```python
from build123d import *

# Parameters (mm, degrees)
SKETCH_281X300_25_R   = 1.6
SKETCH_281X300_25_R_2 = 15
SKETCH_281X300_25_R_3 = 2.15
SKETCH_281X300_25_R_4 = 2.2
SKETCH_281X300_25_W   = 73
SKETCH_281X300_25_H   = 40
F_4MM_DEPTH           = 4
FILLET_1_R            = 8


with BuildPart() as part:
    # Sketch 281x300__25 → 4mm (new body)
    with BuildSketch(Plane.XY):
        Polygon((-51, 150), (53, 150), (53, 100), (137.5, 100), (137.5, -100), (53, -100), (53, -150), (-51, -150), (-51, -100), (-135.5, -100), (-135.5, 100), (-51, 100), align=None)
        with Locations((84.5, -60)):
            Circle(SKETCH_281X300_25_R, mode=Mode.SUBTRACT)
        with Locations((114.5, -60)):
            Circle(SKETCH_281X300_25_R, mode=Mode.SUBTRACT)
        with Locations((84.5, 61)):
            Circle(SKETCH_281X300_25_R, mode=Mode.SUBTRACT)
        with Locations((1, 90.5)):
            Circle(SKETCH_281X300_25_R_2, mode=Mode.SUBTRACT)
        with Locations((1, 125)):
            Circle(SKETCH_281X300_25_R_3, mode=Mode.SUBTRACT)
        with Locations((-33.5, 90.5)):
            Circle(SKETCH_281X300_25_R_3, mode=Mode.SUBTRACT)
        with Locations((35.5, 90.5)):
            Circle(SKETCH_281X300_25_R_3, mode=Mode.SUBTRACT)
        with Locations((-44, 140)):
            Circle(SKETCH_281X300_25_R_3, mode=Mode.SUBTRACT)
        with Locations((114.5, 61)):
            Circle(SKETCH_281X300_25_R, mode=Mode.SUBTRACT)
        with Locations((1, 56)):
            Circle(SKETCH_281X300_25_R_3, mode=Mode.SUBTRACT)
        with Locations((26, -140)):
            Circle(SKETCH_281X300_25_R_4, mode=Mode.SUBTRACT)
        with Locations((-24, -140)):
            Circle(SKETCH_281X300_25_R_4, mode=Mode.SUBTRACT)
        with Locations((-24, -90)):
            Circle(SKETCH_281X300_25_R_4, mode=Mode.SUBTRACT)
        with Locations((26, -90)):
            Circle(SKETCH_281X300_25_R_4, mode=Mode.SUBTRACT)
        with Locations((1, 111.5)):
            Circle(SKETCH_281X300_25_R, mode=Mode.SUBTRACT)
        with Locations((84.5, -90)):
            Circle(SKETCH_281X300_25_R, mode=Mode.SUBTRACT)
        with Locations((84.5, 91)):
            Circle(SKETCH_281X300_25_R, mode=Mode.SUBTRACT)
        with Locations((114.5, 91)):
            Circle(SKETCH_281X300_25_R, mode=Mode.SUBTRACT)
        with Locations((114.5, -90)):
            Circle(SKETCH_281X300_25_R, mode=Mode.SUBTRACT)
        with Locations((118.5, 10)):
            Circle(SKETCH_281X300_25_R, mode=Mode.SUBTRACT)
        with Locations((118.5, -10)):
            Circle(SKETCH_281X300_25_R, mode=Mode.SUBTRACT)
        with Locations((-120.5, 10)):
            Circle(SKETCH_281X300_25_R, mode=Mode.SUBTRACT)
        with Locations((-120.5, -10)):
            Circle(SKETCH_281X300_25_R, mode=Mode.SUBTRACT)
        with Locations((-115.5, -91)):
            Circle(SKETCH_281X300_25_R, mode=Mode.SUBTRACT)
        with Locations((-85.5, -91)):
            Circle(SKETCH_281X300_25_R, mode=Mode.SUBTRACT)
        with Locations((-115.5, 91)):
            Circle(SKETCH_281X300_25_R, mode=Mode.SUBTRACT)
        with Locations((-85.5, 91)):
            Circle(SKETCH_281X300_25_R, mode=Mode.SUBTRACT)
        with Locations((-85.5, 61)):
            Circle(SKETCH_281X300_25_R, mode=Mode.SUBTRACT)
        with Locations((-115.5, 61)):
            Circle(SKETCH_281X300_25_R, mode=Mode.SUBTRACT)
        with Locations((-85.5, -61)):
            Circle(SKETCH_281X300_25_R, mode=Mode.SUBTRACT)
        with Locations((-115.5, -61)):
            Circle(SKETCH_281X300_25_R, mode=Mode.SUBTRACT)
        with Locations((118.5, 43)):
            Circle(SKETCH_281X300_25_R, mode=Mode.SUBTRACT)
        with Locations((118.5, -42)):
            Circle(SKETCH_281X300_25_R, mode=Mode.SUBTRACT)
        with Locations((-120.5, 43)):
            Circle(SKETCH_281X300_25_R, mode=Mode.SUBTRACT)
        with Locations((46, 140)):
            Circle(SKETCH_281X300_25_R_3, mode=Mode.SUBTRACT)
        with Locations((-44, -140)):
            Circle(SKETCH_281X300_25_R_3, mode=Mode.SUBTRACT)
        with Locations((46, -140)):
            Circle(SKETCH_281X300_25_R_3, mode=Mode.SUBTRACT)
        with Locations((19.186533479, 101)):
            Circle(SKETCH_281X300_25_R, mode=Mode.SUBTRACT)
        with Locations((19.186533479, 80)):
            Circle(SKETCH_281X300_25_R, mode=Mode.SUBTRACT)
        with Locations((1, 69.5)):
            Circle(SKETCH_281X300_25_R, mode=Mode.SUBTRACT)
        with Locations((-17.186533479, 80)):
            Circle(SKETCH_281X300_25_R, mode=Mode.SUBTRACT)
        with Locations((-17.186533479, 101)):
            Circle(SKETCH_281X300_25_R, mode=Mode.SUBTRACT)
        with Locations((-120.5, -43)):
            Circle(SKETCH_281X300_25_R, mode=Mode.SUBTRACT)
        with Locations((132.5, 34)):
            Circle(SKETCH_281X300_25_R, mode=Mode.SUBTRACT)
        with Locations((132.5, -73)):
            Circle(SKETCH_281X300_25_R, mode=Mode.SUBTRACT)
        with Locations((72.5, 34)):
            Circle(SKETCH_281X300_25_R, mode=Mode.SUBTRACT)
        with Locations((72.5, -73)):
            Circle(SKETCH_281X300_25_R, mode=Mode.SUBTRACT)
        with Locations((-130.5, 34)):
            Circle(SKETCH_281X300_25_R, mode=Mode.SUBTRACT)
        with Locations((-70.5, 34)):
            Circle(SKETCH_281X300_25_R, mode=Mode.SUBTRACT)
        with Locations((-130.5, -73)):
            Circle(SKETCH_281X300_25_R, mode=Mode.SUBTRACT)
        with Locations((-70.5, -73)):
            Circle(SKETCH_281X300_25_R, mode=Mode.SUBTRACT)
        with BuildLine():
            Line((62.5, -50), (62.5, -36))
            ThreePointArc((62.5, -36), (55, -28.5), (47.5, -36))
            Line((47.5, -36), (47.5, -50))
            ThreePointArc((47.5, -50), (55, -57.5), (62.5, -50))
        make_face(mode=Mode.SUBTRACT)
        with BuildLine():
            Line((-95.5, -10), (-75.5, -10))
            ThreePointArc((-75.5, -10), (-65.5, 0), (-75.5, 10))
            Line((-75.5, 10), (-95.5, 10))
            ThreePointArc((-95.5, 10), (-105.5, 0), (-95.5, -10))
        make_face(mode=Mode.SUBTRACT)
        with Locations((1, -115)):
            Rectangle(SKETCH_281X300_25_W, SKETCH_281X300_25_H, mode=Mode.SUBTRACT)
        with BuildLine():
            Line((47.5, 29), (47.5, 15))
            ThreePointArc((47.5, 15), (55, 7.5), (62.5, 15))
            Line((62.5, 15), (62.5, 29))
            ThreePointArc((62.5, 29), (55, 36.5), (47.5, 29))
        make_face(mode=Mode.SUBTRACT)
    extrude(amount=F_4MM_DEPTH)

    # Fillet 1
    fillet_1_edges = [part.edges().sort_by_distance(p)[0] for p in [
        (53, -150, 2),
        (-51, -150, 2),
        (-51, -100, 2),
        (-135.5, -100, 2),
        (-135.5, 100, 2),
        (-51, 100, 2),
        (-51, 150, 2),
        (53, 150, 2),
        (53, 100, 2),
        (137.5, 100, 2),
        (137.5, -100, 2),
        (53, -100, 2),
        (-35.5, -95, 2),
        (-35.5, -135, 2),
        (37.5, -135, 2),
        (37.5, -95, 2),
    ]]
    fillet(fillet_1_edges, radius=FILLET_1_R)


solid = part.part
```
Can you work these out from the model? Positions are in its coordinate system, mm. A direction names the side the tool comes from. Round coordinates to 2 decimals unless told otherwise and drop trailing zeros. Loops run counter-clockwise (first coordinate to the right, second up) from the corner with the lowest first, then second, coordinate; pieces in that order, holes last.
Item 1: If we mould it in two halves opening along Y, with no side actions, what happens to faces 3 (the flat face through (3, 2, 4)), 4 (the cylindrical face through (54.84, 7.5, 1.97)), 5 (the cylindrical face through (-133.094, 97.719, 2.028)), 6 (the cylindrical face through (-65.5, -0.2, 2))? For each: +Y half, -Y half, draft (parallel to the pull), parting line (faces both ways), or undercut.
Item 2: Please list where these lines run through material, in increasing order: L1, parallel to X at y = 140, z = 1.15; L2, parallel to Y at x = -44, z = 2.85; L3, parallel to Y at x = 26, z = 2.4.
Item 3: Which directions (+Z, -Z, +X, -X, +Y, -Y) give clear straight access to the entire face, cutting with the end or side of a thin tool? Please do faces 1 (the cylindrical face through (55.16, 36.5, 1.97)), 2 (the cylindrical face through (50.719, -147.594, 2.028)).
Item 4: Suppose I cut it at A-A, the plane y = 23. Write out the boundary of the cut face in (x, z), then the cut area to 3 significant figures.
Item 5: Suppose I cut it at C-C, the plane z = 3.2. State how many separate pieces and enclosed holes the cut face has, then the cut area to 3 significant figures.
Item 6: Suppose I cut it at B-B, the plane x = -102. Write out the boundary of the cut face in (y, z).
Item 7: Will these pins go through, and if not, where does the flat tip stop? pin 1 Ø2 at (y, z) = (-114, 2) entering from +X; pin 2 Ø2.5 at (x, y) = (1, 125) entering from -Z.
Reported:
1. face 3: draft
1. face 4: undercut
1. face 5: +Y half
1. face 6: undercut
2. L1: x = -51 to -46.15, -41.85 to 43.85, 48.15 to 53
2. L2: y = -149.94 to -142.15, -137.85 to 137.85, 142.15 to 149.94
2. L3: y = -150 to -142.2, -137.8 to -135, -95 to -92.2, -87.8 to 150
3. face 1: +Z, -Z
3. face 2: +Z, -Z, +X, -Y
4. outline: (-135.5, 0) - (47.5, 0) - (47.5, 4) - (-135.5, 4) - close; (62.5, 0) - (137.5, 0) - (137.5, 4) - (62.5, 4) - close
4. area: 1,030 mm2
5. separate pieces: 1
5. enclosed holes: 55
5. area: 59,400 mm2
6. outline: (-100, 0) - (-7.6, 0) - (-7.6, 4) - (-100, 4) - close; (7.6, 0) - (100, 0) - (100, 4) - (7.6, 4) - close
7. pin 1: stops at x = 53
7. pin 2: passes through
